from build123d import *

# Parameters (mm, degrees)
SKETCH2_W           = 115
SKETCH2_H           = 40
BOSS_EXTRUDE1_DEPTH = 60
CUT_EXTRUDE1_DEPTH  = 60
SKETCH4_R           = 10
CUT_EXTRUDE2_DEPTH  = 60
SKETCH5_W           = 40
SKETCH5_H           = 40
BOSS_EXTRUDE2_DEPTH = 100
SKETCH9_W           = 40
SKETCH9_H           = 100
BOSS_EXTRUDE4_DEPTH = 100
CUT_EXTRUDE10_DEPTH = 100
SKETCH12_W          = 40
SKETCH12_H          = 40
BOSS_EXTRUDE6_DEPTH = 30


with BuildPart() as part:
    # Sketch2 → Boss-Extrude1 (new body)
    with BuildSketch(Plane.XY):
        with Locations((-2.12962963, 23.505291005)):
            Rectangle(SKETCH2_W, SKETCH2_H)
    extrude(amount=BOSS_EXTRUDE1_DEPTH)

    # Sketch3 → Cut-Extrude1 (cut)
    with BuildSketch(Plane(origin=(0, 43.505291005, 0), x_dir=(1, 0, 0), z_dir=(0, 1, 0))):
        with BuildLine():
            Line((-59.62962963, -30), (-24.62962963, -30))
            ThreePointArc((-24.62962963, -30), (-2.12962963, -7.5), (20.37037037, -30))
            Line((20.37037037, -30), (55.37037037, -30))
            Line((55.37037037, -30), (55.37037037, -60))
            Line((55.37037037, -60), (-59.62962963, -60))
            Line((-59.62962963, -60), (-59.62962963, -30))
        make_face()
    extrude(amount=-CUT_EXTRUDE1_DEPTH, mode=Mode.SUBTRACT)

    # Sketch4 → Cut-Extrude2 (cut)
    with BuildSketch(Plane.XY.offset(30)):
        with Locations((-42.12962963, 23.505291005)):
            Circle(SKETCH4_R)
        with Locations((37.87037037, 23.505291005)):
            Circle(SKETCH4_R)
    extrude(amount=-CUT_EXTRUDE2_DEPTH, mode=Mode.SUBTRACT)

    # Sketch5 → Boss-Extrude2 (add)
    with BuildSketch(Plane(origin=(0, 0, 0), x_dir=(-1, 0, 0), z_dir=(0, 0, -1))):
        with Locations((2.12962963, 23.505291005)):
            Rectangle(SKETCH5_W, SKETCH5_H)
    extrude(amount=BOSS_EXTRUDE2_DEPTH)

    # Sketch9 → Boss-Extrude4 (add)
    with BuildSketch(Plane(origin=(0, 43.505291005, 0), x_dir=(1, 0, 0), z_dir=(0, 1, 0))):
        with Locations((-2.12962963, 50)):
            Rectangle(SKETCH9_W, SKETCH9_H)
    extrude(amount=BOSS_EXTRUDE4_DEPTH)

    # Sketch10 → Cut-Extrude10 (cut)
    with BuildSketch(Plane(origin=(17.87037037, 0, 0), x_dir=(0, 0, -1), z_dir=(1, 0, 0))):
        Polygon((100, 43.505291005), (29.289321881, 114.215969124), (29.289321881, 94.215969124), (80, 43.505291005), (0, 43.505291005), (0, 143.505291005), (100, 143.505291005), align=None)
    extrude(amount=-CUT_EXTRUDE10_DEPTH, mode=Mode.SUBTRACT)

    # Sketch12 → Boss-Extrude6 (add)
    with BuildSketch(Plane(origin=(0, 71.752645503, -71.752645503), x_dir=(1, 0, 0), z_dir=(0, 0.7071067811865513, -0.7071067811865438))):
        with Locations((-2.12962963, -30.052208169)):
            Rectangle(SKETCH12_W, SKETCH12_H)
    extrude(amount=BOSS_EXTRUDE6_DEPTH)


solid = part.part
Check sheet for the modelled part. Datum: model origin and axes. Units: mm. A direction names the side the tool comes from. Give positions to 0.01 mm unless a question says otherwise; leave off trailing zeros. Order: outer loops, then holes, each group sorted by start corner. A loop starts at its lowest first (then second) coordinate and runs counter-clockwise, first axis right, second up. Notation, with made-up numbers: (59.25, 62) - (111.25, 62) arc R16 ccw to (111.25, 83) - close; hole circle Ø2 at (-10.75, 62). An arc over 180 degrees is marked (long way). Answer as CSV lines item,"result".
1. Section check B-B (y = 19.5). Record the boundary of the cut face in (x, z), then the cut area to 3 significant figures.
Result sheet:
outline,"(-59.63, 0) - (-51.29, 0) - (-51.29, 30) - (-59.63, 30) - close; (-32.97, 0) - (-22.13, 0) - (-22.13, -100) - (17.87, -100) - (17.87, 0) - (28.71, 0) - (28.71, 30) - (20.37, 30) arc R22.5 cw to (-24.63, 30) - (-32.97, 30) - close; (47.03, 0) - (55.37, 0) - (55.37, 30) - (47.03, 30) - close"
area,"5,560 mm²"
2. Tool access check on faces 4 (the face through (28, 28, 0)), 5 (the face through (-33, 28, 0)), 6 (the face through (-1.85, 110.631, -32.874)), 7 (the face through (-1, 43.505, -14)). Record the directions out of +Z, -Z, +X, -X, +Y, -Y that give a thin tool (end or side, any length) a straight path to the whole face; none if there is none.
Result sheet:
face 4,"-Z, +X, +Y, -Y"
face 5,"-Z, -X, +Y, -Y"
face 6,"+X, -X, +Y"
face 7,"+Z, +X, -X"
3. Scan lines: probe 1 along X at (y, z) = (58, -74); probe 2 along Y at (x, z) = (-16.5, -21.5); probe 3 along Z at (x, y) = (49.5, 41.5). Record each from-to range of solid material in increasing order. Write a range as from..to.
Result sheet:
probe 1,"-22.13..17.87"
probe 2,"3.51..43.51"
probe 3,"0..30"
4. Section check A-A (z = -47). Record the boundary of the cut face in (x, y), then the cut area to 3 significant figures.
Result sheet:
outline,"(-22.13, 3.51) - (17.87, 3.51) - (17.87, 43.51) - (-22.13, 43.51) - close; (-22.13, 76.51) - (17.87, 76.51) - (17.87, 117.78) - (-22.13, 117.78) - close"
area,"3,250 mm²"
5. Mould release check, pull along X, two halves, no side actions. Record for faces 1 (the face through (-2.41, 117.603, -46.818)), 2 (the face through (-22.13, 37, -49)), 3 (the face through (-2.624, 23.785, 7.505)): released by +X, released by -X, zero draft, split by the parting line, or undercut.
Result sheet:
face 1,"zero draft"
face 2,"released by -X"
face 3,"undercut"
6. Section check C-C (y = 39). Record the boundary of the cut face in (x, z), then the cut area to 3 significant figures.
Result sheet:
outline,"(-59.63, 0) - (-22.13, 0) - (-22.13, -100) - (17.87, -100) - (17.87, 0) - (55.37, 0) - (55.37, 30) - (20.37, 30) arc R22.5 cw to (-24.63, 30) - (-59.63, 30) - close"
area,"6,650 mm²"
7. Section check D-D (x = -47). Record the boundary of the cut face in (y, z).
Result sheet:
outline,"(3.51, 0) - (14.77, 0) - (14.77, 30) - (3.51, 30) - close; (32.24, 0) - (43.51, 0) - (43.51, 30) - (32.24, 30) - close"
8. Go/stop test with flat-tipped pins: P1, Ø19, axis at x = -40.5, y = 16.5, coming from the -Z side; P2, Ø10, axis at x = 13, z = -13, coming from the +Y side; P3, Ø8, axis at x = -3, z = -45.5, coming from the +Y side. Record where each tip stops, or that it passes through.
Result sheet:
P1,"z = 0"
P2,"y = 43.51"
P3,"y = 120.28"
